Can you work these out from the drawing? Everything is in mm from the part's minimum corner. A direction names the side the tool comes from. Give positions to 0.01 mm unless a question says otherwise; leave off trailing zeros. Loops run counter-clockwise (first coordinate to the right, second up) from the corner with the lowest first, then second, coordinate; pieces in that order, holes last. Notation, with made-up numbers: (42.5, -8) - (79.5, -8) arc R19 ccw to (79.5, 25) - close; hole circle Ø9 at (8, -5). An arc over 180 degrees is marked (long way). One line per item, written item: value. Start each with the question number.
Q1. I want a section at A-A (x = 27). Please give me the cut outline in (y, z) (1 decimal), then the cut area to 3 significant figures.
Q2. I want a section at B-B (z = 31.5). Please give me the cut outline in (x, y).
Q3. I want a section at D-D (y = 9.5). Please give me the cut outline in (x, z) (1 decimal).
Q4. I want a section at C-C (x = 19.5). Please give me the cut outline in (y, z).
Q5. I'm going to push flat-ended pins straight in: P1, Ø8, axis at x = 33, z = 14, coming from the -Y side; P2, Ø1.5, axis at x = 29, y = 7.5, coming from the +Z side (1 decimal); P3, Ø5, axis at y = 5, z = 22, coming from the -X side. Where does each tip first touch, or does it pass through?
Q6. If I drill on line 1 (X direction, y = 30.5, z = 32.5); line 2 (Z direction, x = 26, y = 44); line 3 (Y direction, x = 33.5, z = 42.5), over which ranges is the centre line in solid material (lowest first)? Write a range as from..to.
Q7. For the marked faces 1 and 2, which set-ups out of +Z, -Z, +X, -X, +Y, -Y let a thin tool reach every point of the face, with its end or its side?
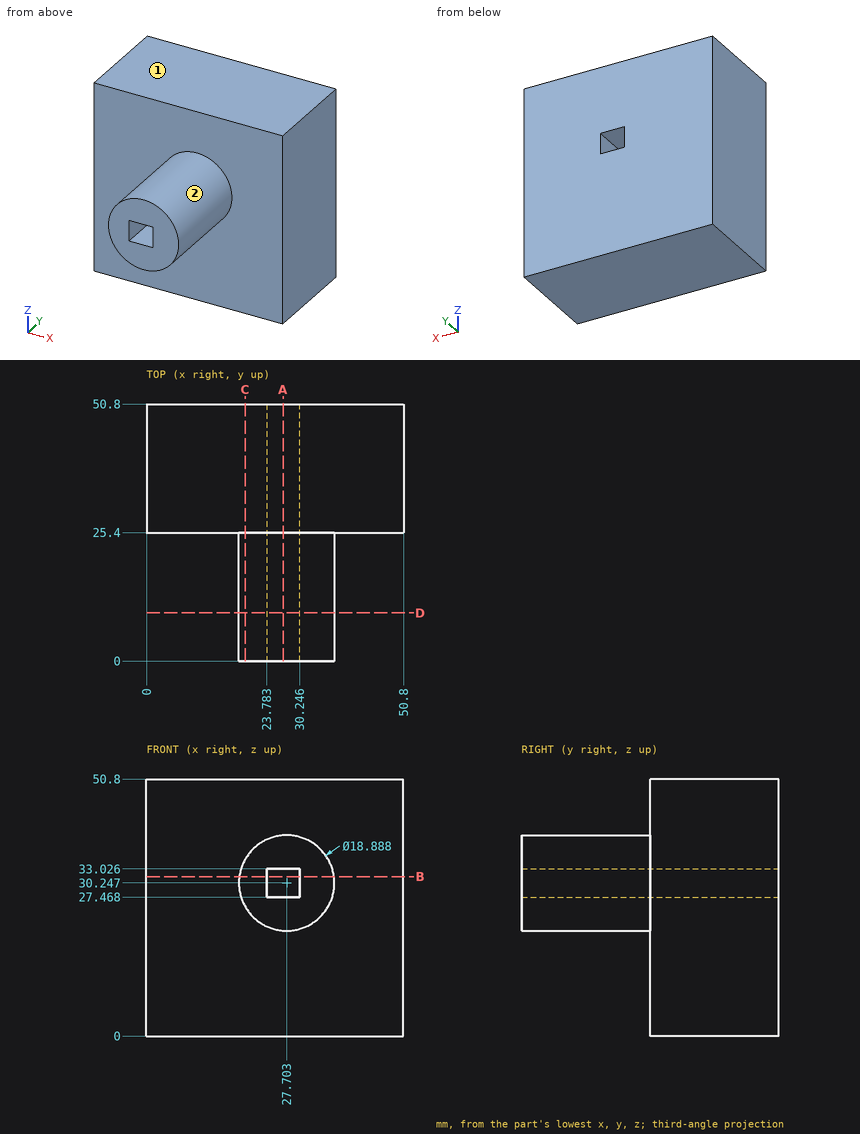
Worked answers:
1. outline: (0, 20.8) - (25.4, 20.8) - (25.4, 0) - (50.8, 0) - (50.8, 27.5) - (0, 27.5) - close; (0, 33) - (50.8, 33) - (50.8, 50.8) - (25.4, 50.8) - (25.4, 39.7) - (0, 39.7) - close
1. area: 1,490 mm²
2. outline: (0, 25.4) - (18.34, 25.4) - (18.34, 0) - (23.78, 0) - (23.78, 50.8) - (0, 50.8) - close; (30.25, 0) - (37.06, 0) - (37.06, 25.4) - (50.8, 25.4) - (50.8, 50.8) - (30.25, 50.8) - close
3. outline: circle Ø18.9 at (27.7, 30.2); hole (23.8, 27.5) - (30.2, 27.5) - (30.2, 33) - (23.8, 33) - close
4. outline: (0, 25.57) - (25.4, 25.57) - (25.4, 0) - (50.8, 0) - (50.8, 50.8) - (25.4, 50.8) - (25.4, 34.93) - (0, 34.93) - close
5. P1: stops at y = 25.4
5. P2: stops at z = 39.7
5. P3: stops at x = 20.21
6. line 1: x = 0..23.78, 30.25..50.8
6. line 2: z = 0..27.47, 33.03..50.8
6. line 3: y = 25.4..50.8
7. face 1: +Z, +X, -X, +Y, -Y
7. face 2: -Y
